For this review, use the dimensioned drawing (mm, ordinates from the lowest corner) and the shaded views. Round coordinates to 2 decimals unless told otherwise and drop trailing zeros. Loops run counter-clockwise (first coordinate to the right, second up) from the corner with the lowest first, then second, coordinate; pieces in that order, holes last. Notation, with made-up numbers: (-28, 14) - (-20, 14) arc R20 ccw to (-20, 18) - close; hole circle Ø1 at (-5.5, 71). An arc over 180 degrees is marked (long way). Answer as CSV lines item,"result". Start each with the question number.
(1) Consider section B-B (z = 10). Give the boundary of the cut face in (x, y), and give its area (3 significant figures).
(2) Consider section D-D (z = 29). Give the boundary of the cut face in (x, y), and give its area (3 significant figures).
(3) For P1, Ø1.5, axis at x = 1.5, y = 28.5, coming from the -Z side; P2, Ø1.5, axis at x = 1, y = 46, coming from the +Z side; P3, Ø1.5, axis at x = 2, y = 24.5, coming from the -Z side, all flat-tipped, find the tip position at first contact; note any pin that passes through.
(4) Wall thickness on L1, parallel to Y at x = 1.95, z = 30; L2, parallel to Y at x = 1.3, z = 50; L3, parallel to Y at x = 1.4, z = 55: over which ranges is each line inside the solid? List them lowest first.
(5) Consider section A-A (y = 50). Give the boundary of the cut face in (x, z), and give its area (3 significant figures).
(6) Consider section C-C (x = 1.85). Give the boundary of the cut face in (y, z), and give its area (3 significant figures).
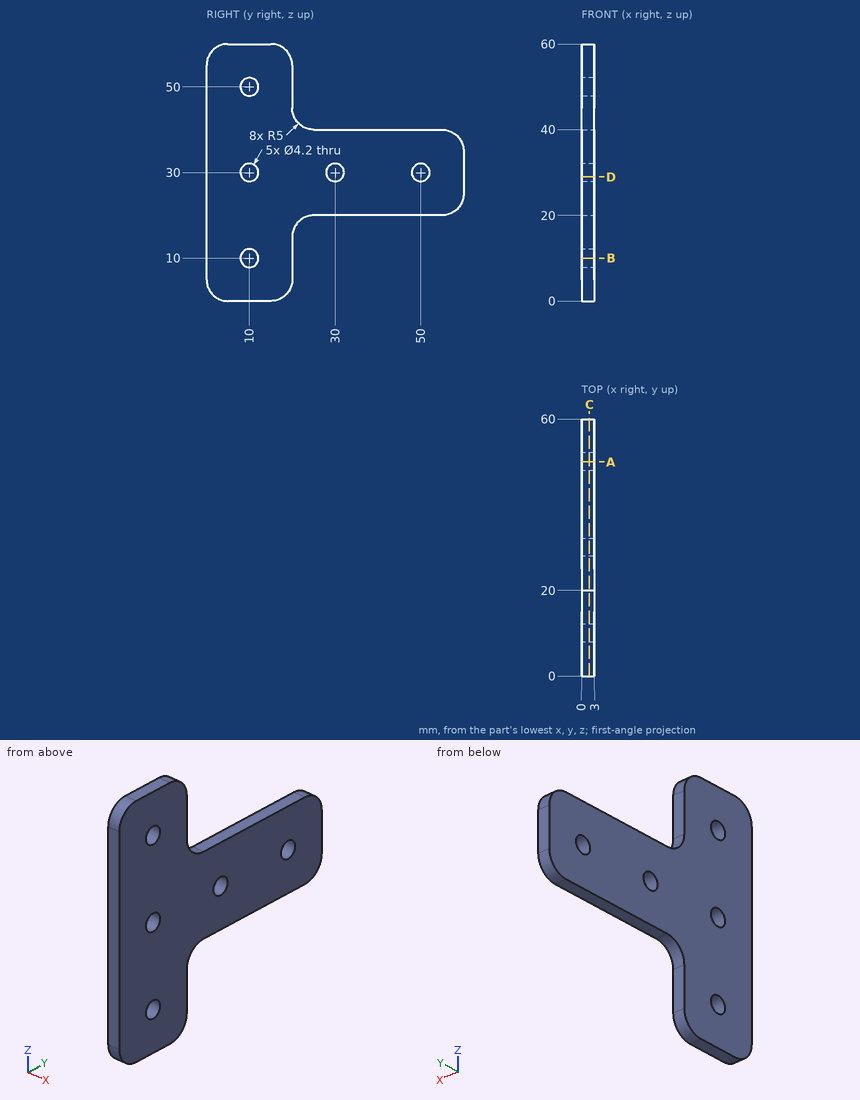
Determined:
1,outline,"(0, 0) - (3, 0) - (3, 7.9) - (0, 7.9) - close; (0, 12.1) - (3, 12.1) - (3, 20) - (0, 20) - close"
1,area,"47.4 mm^2"
2,outline,"(0, 0) - (3, 0) - (3, 8.15) - (0, 8.15) - close; (0, 11.85) - (3, 11.85) - (3, 28.15) - (0, 28.15) - close; (0, 31.85) - (3, 31.85) - (3, 48.15) - (0, 48.15) - close; (0, 51.85) - (3, 51.85) - (3, 60) - (0, 60) - close"
2,area,"147 mm^2"
3,P1,"stops at z = 20"
3,P2,"stops at z = 40"
3,P3,"stops at z = 19.84"
4,L1,"y = 0 to 7.9, 12.1 to 27.9, 32.1 to 47.9, 52.1 to 60"
4,L2,"y = 0 to 7.9, 12.1 to 20"
4,L3,"y = 0 to 20"
5,outline,"(0, 20) - (3, 20) - (3, 27.9) - (0, 27.9) - close; (0, 32.1) - (3, 32.1) - (3, 40) - (0, 40) - close"
5,area,"47.4 mm^2"
6,outline,"(0, 5) arc R5 ccw to (5, 0) - (15, 0) arc R5 ccw to (20, 5) - (20, 15) arc R5 cw to (25, 20) - (55, 20) arc R5 ccw to (60, 25) - (60, 35) arc R5 ccw to (55, 40) - (25, 40) arc R5 cw to (20, 45) - (20, 55) arc R5 ccw to (15, 60) - (5, 60) arc R5 ccw to (0, 55) - close; hole circle Ø4.2 at (10, 10); hole circle Ø4.2 at (10, 30); hole circle Ø4.2 at (10, 50); hole circle Ø4.2 at (30, 30); hole circle Ø4.2 at (50, 30)"
6,area,"1,910 mm^2"
